from build123d import *

# Parameters (mm, degrees)
BOSS_EXTRUDE1_DEPTH = 1.524


with BuildPart() as part:
    # Sketch1 → Boss-Extrude1 (new body)
    with BuildSketch(Plane.XY):
        with BuildLine():
            Line((1.507959842, 1.524), (1.507959842, 0))
            Line((1.507959842, 0), (3.052407177, 0))
            Line((3.052407177, 0), (3.052407177, -1.566256329))
            ThreePointArc((3.052407177, -1.566256329), (-0.719055485, -5.336831222), (-5.053668942, -8.443644993))
            ThreePointArc((-5.053668942, -8.443644993), (-14.427584678, -14.984368639), (-21.770031842, -23.744496018))
            ThreePointArc((-21.770031842, -23.744496018), (-17.037991297, -15.548436862), (-9.89443504, -9.340603312))
            ThreePointArc((-9.89443504, -9.340603312), (-7.376811542, -7.92151996), (-5.053668942, -6.202440528))
            ThreePointArc((-5.053668942, -6.202440528), (-3.071218913, -3.363942956), (-2.252033724, 0))
            Line((-2.252033724, 0), (-2.252033724, 1.524))
            Line((-2.252033724, 1.524), (1.507959842, 1.524))
        make_face()
    extrude(amount=BOSS_EXTRUDE1_DEPTH)


solid = part.part
Work out the finished part from the listing and answer in its coordinate system (mm). A direction names the side the tool comes from. Round coordinates to 2 decimals unless told otherwise and drop trailing zeros. Loops run counter-clockwise (first coordinate to the right, second up) from the corner with the lowest first, then second, coordinate; pieces in that order, holes last. Notation, with made-up numbers: (72, -8.75) -> (109, -8.75) arc R23 cw to (109, 12.25) -> close; hole circle Ø1 at (-5, 53). An arc over 180 degrees is marked (long way). Use one line per item in the form item = value.
(1) Find section B-B on x = -2.75. Give the vertices of the cut face in (y, z).
Answer list:
outline = (-6.93, 0) -> (-2.55, 0) -> (-2.55, 1.52) -> (-6.93, 1.52) -> close
(2) Find section A-A on z = 1.1. Give the vertices of the cut face in (x, y), then the cut area to 3 significant figures.
Answer list:
outline = (-21.77, -23.74) arc R43.42 cw to (-5.05, -8.44) arc R32.67 ccw to (3.05, -1.57) -> (3.05, 0) -> (1.51, 0) -> (1.51, 1.52) -> (-2.25, 1.52) -> (-2.25, 0) arc R9.39 cw to (-5.05, -6.2) arc R23.36 cw to (-9.89, -9.34) arc R28.66 ccw to start
area = 68.8 mm2
(3) Find section C-C on y = -17. Give the vertices of the cut face in (x, z).
Answer list:
outline = (-18.16, 0) -> (-16.49, 0) -> (-16.49, 1.52) -> (-18.16, 1.52) -> close
(4) A tool of negligible diameter and unlimited length cuts with its end or side. For faces 1 (the flat face through (2, 0, 1)), 2 (the cylindrical face through (-14.309, -14.876, 0.751)), 3 (the flat face through (-2.252, 1, 1)), from which of +Z, -Z, +X, -X, +Y, -Y can it reach the whole face along a straight path? Write none if from no direction.
Answer list:
face_1 = +Z, -Z, +X, +Y
face_2 = +Z, -Z, +X, -Y
face_3 = +Z, -Z, -X, +Y
(5) Straight lines are drawn through the part: line 1 (Y direction, x = -13, z = 0.6); line 2 (Y direction, x = -12.25, z = 0.2); line 3 (X direction, y = -14.25, z = 0.55). For each, find the intervals that lie inside material, in ascending order.
Answer list:
line_1 = -13.73 to -11.54
line_2 = -13.12 to -10.95
line_3 = -15.9 to -13.6
(6) Flat-ended cylindrical pins translate along their axes: P1, Ø0.8, axis at x = 2, z = 0.5, coming from the +Y side; P2, Ø0.5, axis at y = 1, z = 0.5, coming from the -X side. Find the tip coordinate at first contact, or state that the pin passes through.
Answer list:
P1 = 0
P2 = -2.25
